```python
from build123d import *

# Parameters (mm, degrees)
CHAMFER_1_SIZE       = 0.5
SKETCH_2_OUTSIDE_W   = 90.032
SKETCH_2_OUTSIDE_H   = 90.032
SKETCH_2_OUTSIDE_W_2 = 7
SKETCH_2_OUTSIDE_H_2 = 8
CUT_EXTRUDE_1_DEPTH  = 8


with BuildPart() as part:
    # 草图1 → 旋转1 (revolve)
    with BuildSketch(Plane.XY, mode=Mode.PRIVATE) as revolve_1_sk:
        Polygon((-200, 2.15), (-190, 2.15), (-188.708149669, 0), (188.708149669, 0), (190, 2.15), (200, 2.15), (200, 4), (-200, 4), align=None)
    revolve(revolve_1_sk.sketch.rotate(Axis((0, 0, 0), (1, 0, 0)), 90), axis=Axis((0, 0, 0), (1, 0, 0)))

    # 倒角1
    chamfer_1_edges = [part.edges().sort_by_distance(p)[0] for p in [
        (-200, 0, -4),
        (200, 0, -4),
    ]]
    chamfer(chamfer_1_edges, length=CHAMFER_1_SIZE)

    # 草图2 outside → 切除-拉伸1 (cut)
    with BuildSketch(Plane.ZY.offset(140)):
        Rectangle(SKETCH_2_OUTSIDE_W, SKETCH_2_OUTSIDE_H)
        Rectangle(SKETCH_2_OUTSIDE_W_2, SKETCH_2_OUTSIDE_H_2, mode=Mode.SUBTRACT)
    extrude(amount=-CUT_EXTRUDE_1_DEPTH, mode=Mode.SUBTRACT)


solid = part.part
```
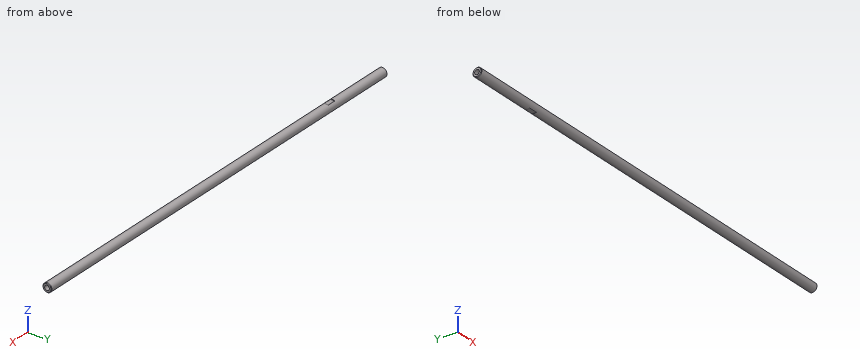
Work out the finished part from the listing and answer in its coordinate system (mm). Coordinates: 2 decimals unless noted, no trailing zeros. Loops run counter-clockwise (first coordinate to the right, second up) from the corner with the lowest first, then second, coordinate; pieces in that order, holes last.
1) Flat-ended cylindrical pins translate along their axes: pin 1 (2 mm diameter, centred on x = 45, z = 1.5, fed in from +Y); pin 2 (4 mm diameter, centred on y = -1, z = -1.5, fed in from +X); pin 3 (1.5 mm diameter, centred on y = -0.5, z = -1, fed in from +X); pin 4 (1 mm diameter, centred on x = 144, y = 2, fed in from -Z). Find the tip coordinate at first contact, or state that the pin passes through.
Results:
pin 1: stops at y = 3.97
pin 2: stops at x = 200
pin 3: stops at x = 189.83
pin 4: stops at z = -3.71
2) Section A-A (x = 101) is taken. Give the vertices of the cut face in (y, z).
Results:
outline: circle Ø8 at (0, 0)
3) Consider probe 1 along Y at (x, z) = (-194, 0); probe 2 along Y at (x, z) = (-54, 3.5); probe 3 along X at (y, z) = (2.5, -2.5). Determine where each line is inside the solid, lowest interval first.
Results:
probe 1: y = -4 to -2.15, 2.15 to 4
probe 2: y = -1.94 to 1.94
probe 3: x = -199.96 to 199.96
